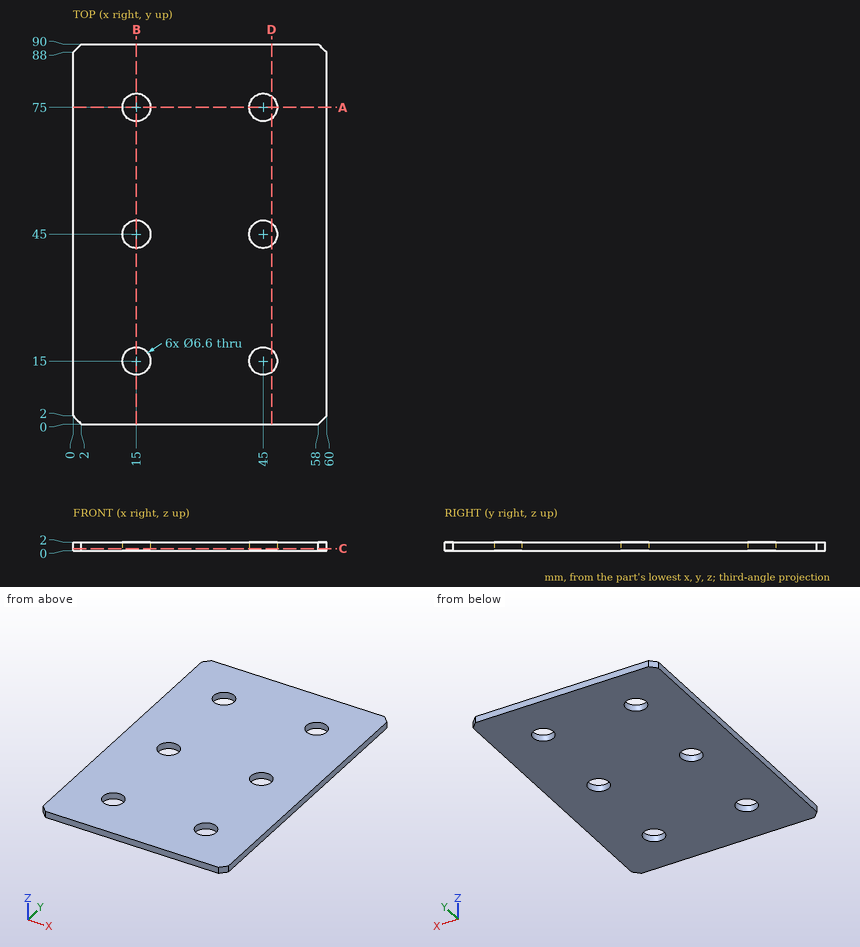
For this review, use the dimensioned drawing (mm, ordinates from the lowest corner) and the shaded views. Give positions to 0.01 mm unless a question says otherwise; leave off trailing zeros. Order: outer loops, then holes, each group sorted by start corner. A loop starts at its lowest first (then second) coordinate and runs counter-clockwise, first axis right, second up.
1. Add section B-B, the plane x = 15. State the section outline as (y, z) points, then the cut area to 3 significant figures.
Solution:
outline: (0, 0) - (11.7, 0) - (11.7, 2) - (0, 2) - close; (18.3, 0) - (41.7, 0) - (41.7, 2) - (18.3, 2) - close; (48.3, 0) - (71.7, 0) - (71.7, 2) - (48.3, 2) - close; (78.3, 0) - (90, 0) - (90, 2) - (78.3, 2) - close
area: 140 mm2
2. Add section A-A, the plane y = 75. State the section outline as (x, z) points, then the cut area to 3 significant figures.
Solution:
outline: (0, 0) - (11.7, 0) - (11.7, 2) - (0, 2) - close; (18.3, 0) - (41.7, 0) - (41.7, 2) - (18.3, 2) - close; (48.3, 0) - (60, 0) - (60, 2) - (48.3, 2) - close
area: 93.6 mm2
3. To check wall thickness, follow L1, parallel to Y at x = 45, z = 0.5; L2, parallel to X at y = 46.5, z = 1.6; L3, parallel to Y at x = 14, z = 0.15. State the ranges of each line that lie inside material, in increasing order.
Solution:
L1: y = 0 to 11.7, 18.3 to 41.7, 48.3 to 71.7, 78.3 to 90
L2: x = 0 to 12.06, 17.94 to 42.06, 47.94 to 60
L3: y = 0 to 11.86, 18.14 to 41.86, 48.14 to 71.86, 78.14 to 90
4. For pin 1 Ø6 at (x, y) = (15, 75) entering from +Z, flat-tipped, find the tip position at first contact; note if it passes through.
Solution:
pin 1: passes through
5. Add section D-D, the plane x = 47. State the section outline as (y, z) points.
Solution:
outline: (0, 0) - (12.38, 0) - (12.38, 2) - (0, 2) - close; (17.62, 0) - (42.38, 0) - (42.38, 2) - (17.62, 2) - close; (47.62, 0) - (72.38, 0) - (72.38, 2) - (47.62, 2) - close; (77.62, 0) - (90, 0) - (90, 2) - (77.62, 2) - close
6. Add section C-C, the plane z = 0.5. State the section outline as (x, y) points, then the cut area to 3 significant figures.
Solution:
outline: (0, 2) - (2, 0) - (58, 0) - (60, 2) - (60, 88) - (58, 90) - (2, 90) - (0, 88) - close; hole circle Ø6.6 at (15, 15); hole circle Ø6.6 at (15, 45); hole circle Ø6.6 at (15, 75); hole circle Ø6.6 at (45, 15); hole circle Ø6.6 at (45, 45); hole circle Ø6.6 at (45, 75)
area: 5,190 mm2
